Input: part model. Units: mm. Frame: model coordinates. Give positions to 0.01 mm unless a question says otherwise; leave off trailing zeros. Loops run counter-clockwise (first coordinate to the right, second up) from the corner with the lowest first, then second, coordinate; pieces in that order, holes last.
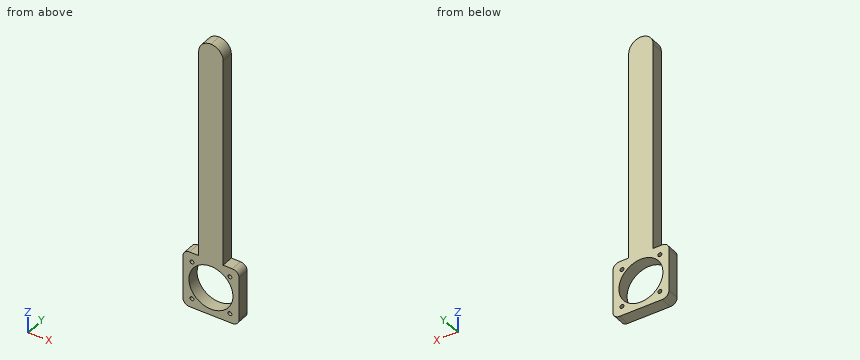
from build123d import *

# Parameters (mm, degrees)
SKETCH_2_W          = 46
SKETCH_2_H          = 46
SKETCH_2_R          = 18
EXTRUDE_1_DEPTH     = 10
FILLET_1_R          = 5.5
SKETCH_3_R          = 1.6
CUT_EXTRUDE_1_DEPTH = 35.029399054
SKETCH_4_W          = 20
SKETCH_4_H          = 182
EXTRUDE_2_DEPTH     = 10
FILLET_2_R          = 10


with BuildPart() as part:
    # 草图2 → 凸台-拉伸1 (new body)
    with BuildSketch(Plane(origin=(0, 0, 0), x_dir=(1, 0, 0), z_dir=(0, 1, 0))):
        Rectangle(SKETCH_2_W, SKETCH_2_H)
        with Locations(Location((0, 0, 0), (0, 0, 270))):
            Circle(SKETCH_2_R, mode=Mode.SUBTRACT)
    extrude(amount=EXTRUDE_1_DEPTH)

    # 圆角1
    fillet_1_edges = [part.edges().sort_by_distance(p)[0] for p in [
        (23, 5, 23),
        (-23, 5, 23),
        (-23, 5, -23),
        (23, 5, -23),
    ]]
    fillet(fillet_1_edges, radius=FILLET_1_R)

    # 草图3 → 切除-拉伸1 (cut, through all)
    with BuildSketch(Plane(origin=(0, 10, 0), x_dir=(1, 0, 0), z_dir=(0, 1, 0))):
        with Locations(Location((-15.5, 15.5, 0), (0, 0, 270))):
            Circle(SKETCH_3_R)
        with Locations(Location((15.5, 15.5, 0), (0, 0, 270))):
            Circle(SKETCH_3_R)
        with Locations(Location((-15.5, -15.5, 0), (0, 0, 270))):
            Circle(SKETCH_3_R)
        with Locations(Location((15.5, -15.5, 0), (0, 0, 270))):
            Circle(SKETCH_3_R)
    extrude(amount=-CUT_EXTRUDE_1_DEPTH, mode=Mode.SUBTRACT)

    # 草图4 → 凸台-拉伸2 (add)
    with BuildSketch(Plane(origin=(0, 10, 0), x_dir=(1, 0, 0), z_dir=(0, 1, 0))):
        with Locations((0, -114)):
            Rectangle(SKETCH_4_W, SKETCH_4_H)
    extrude(amount=-EXTRUDE_2_DEPTH)

    # 圆角2
    fillet_2_edges = [part.edges().sort_by_distance(p)[0] for p in [
        (-10, 5, 205),
        (10, 5, 205),
    ]]
    fillet(fillet_2_edges, radius=FILLET_2_R - 0.0001)  # a hair under: the kernel refuses the full size


solid = part.part
(1) Cut plane A-A (z = 0). Return the cut outline in (x, y), and give its area (3 significant figures).
Values follow:
outline: (-23, 0) - (-18, 0) - (-18, 10) - (-23, 10) - close; (18, 0) - (23, 0) - (23, 10) - (18, 10) - close
area: 100 mm2
(2) Cut plane B-B (y = 6.25). Count the separate pieces of the cut face and the enclosed holes in it, and give its area (3 significant figures).
Values follow:
separate pieces: 1
enclosed holes: 5
area: 4,640 mm2
(3) Cut plane D-D (z = 117). Return the cut outline in (x, y).
Values follow:
outline: (-10, 0) - (10, 0) - (10, 10) - (-10, 10) - close
(4) Cut plane C-C (x = -4.5). Return the cut outline in (y, z).
Values follow:
outline: (0, -23) - (10, -23) - (10, -17.43) - (0, -17.43) - close; (0, 17.43) - (10, 17.43) - (10, 203.93) - (0, 203.93) - close
(5) Ray query, probe 1 along Z at (x, y) = (-16, 8.75); probe 2 along X at (y, z) = (4, 15.5); probe 3 along Z at (x, y) = (0.5, 6.5). Return the intervals inside material, ascending.
Values follow:
probe 1: z = -23 to -17.02, -13.98 to -8.25, 8.25 to 13.98, 17.02 to 23
probe 2: x = -23 to -17.1, -13.9 to -9.15, 9.15 to 13.9, 17.1 to 23
probe 3: z = -23 to -17.99, 17.99 to 204.99
(6) Pin query (flat end, axial travel): pin 1 Ø1.5 at (y, z) = (3.5, 144) entering from -X; pin 2 Ø6 at (x, y) = (18, 2) entering from +Z. Return the tip coordinate at first contact, or that it passes through.
Values follow:
pin 1: stops at x = -10
pin 2: stops at z = 23
